Check sheet for the modelled part. Datum: model origin and axes. Units: mm. A direction names the side the tool comes from. Give positions to 0.01 mm unless a question says otherwise; leave off trailing zeros. Write each loop counter-clockwise with the first axis right and the second up, starting at its lowest first coordinate (ties: lowest second). Pieces come first, ordered by that corner, then holes. Notation, with made-up numbers: (75, 30) -> (115, 30) arc R18 ccw to (115, 52) -> close; hole circle Ø3 at (-15.75, -26). An arc over 180 degrees is marked (long way). Answer as a JSON object with one key per item and string values.
from build123d import *

# Parameters (mm, degrees)
SKETCH1_R           = 1.6
BOSS_EXTRUDE1_DEPTH = 7.5


with BuildPart() as part:
    # Sketch1 → Boss-Extrude1 (new body)
    with BuildSketch(Plane(origin=(0, 0, 0), x_dir=(1, 0, 0), z_dir=(0, 1, 0))):
        with BuildLine():
            Line((-5, 43.966606646), (-5, 44.520107817))
            ThreePointArc((-5, 44.520107817), (0, 44.8), (5, 44.520107817))
            Line((5, 44.520107817), (5, 43.966606646))
            ThreePointArc((5, 43.966606646), (31.289475068, 31.289475068), (43.966606646, 5))
            Line((43.966606646, 5), (44.520107817, 5))
            ThreePointArc((44.520107817, 5), (44.8, 0), (44.520107817, -5))
            Line((44.520107817, -5), (43.966606646, -5))
            ThreePointArc((43.966606646, -5), (31.289475068, -31.289475068), (5, -43.966606646))
            Line((5, -43.966606646), (5, -44.520107817))
            ThreePointArc((5, -44.520107817), (0, -44.8), (-5, -44.520107817))
            Line((-5, -44.520107817), (-5, -43.966606646))
            ThreePointArc((-5, -43.966606646), (-31.289475068, -31.289475068), (-43.966606646, -5))
            Line((-43.966606646, -5), (-44.520107817, -5))
            ThreePointArc((-44.520107817, -5), (-44.8, 0), (-44.520107817, 5))
            Line((-44.520107817, 5), (-43.966606646, 5))
            ThreePointArc((-43.966606646, 5), (-31.289475068, 31.289475068), (-5, 43.966606646))
        make_face()
        with Locations(Location((36.25, 0, 0), (0, 0, 270))):
            Circle(SKETCH1_R, mode=Mode.SUBTRACT)
        with Locations(Location((0, -36.25, 0), (0, 0, 270))):
            Circle(SKETCH1_R, mode=Mode.SUBTRACT)
        with Locations(Location((-36.25, 0, 0), (0, 0, 270))):
            Circle(SKETCH1_R, mode=Mode.SUBTRACT)
        with Locations(Location((0, 36.25, 0), (0, 0, 270))):
            Circle(SKETCH1_R, mode=Mode.SUBTRACT)
        with BuildLine():
            Line((33.430226046, 5), (36.586370413, 5))
            ThreePointArc((36.586370413, 5), (38.127746073, 5.725574218), (38.550739294, 7.375838926))
            ThreePointArc((38.550739294, 7.375838926), (36.262271651, 15.02032472), (32.474994896, 22.043983453))
            ThreePointArc((32.474994896, 22.043983453), (21.567115852, 32.79362764), (7.375838926, 38.550739294))
            ThreePointArc((7.375838926, 38.550739294), (5.725574218, 38.127746073), (5, 36.586370413))
            Line((5, 36.586370413), (5, 33.430226046))
            ThreePointArc((5, 33.430226046), (4.414213562, 32.016012484), (3, 31.430226046))
            Line((3, 31.430226046), (-3, 31.430226046))
            ThreePointArc((-3, 31.430226046), (-4.414213562, 32.016012484), (-5, 33.430226046))
            Line((-5, 33.430226046), (-5, 36.586370413))
            ThreePointArc((-5, 36.586370413), (-5.725574218, 38.127746073), (-7.375838926, 38.550739294))
            ThreePointArc((-7.375838926, 38.550739294), (-27.753941162, 27.753941162), (-38.550739294, 7.375838926))
            ThreePointArc((-38.550739294, 7.375838926), (-38.127746073, 5.725574218), (-36.586370413, 5))
            Line((-36.586370413, 5), (-33.430226046, 5))
            ThreePointArc((-33.430226046, 5), (-32.016012484, 4.414213562), (-31.430226046, 3))
            Line((-31.430226046, 3), (-31.430226046, -3))
            ThreePointArc((-31.430226046, -3), (-32.016012484, -4.414213562), (-33.430226046, -5))
            Line((-33.430226046, -5), (-36.586370413, -5))
            ThreePointArc((-36.586370413, -5), (-38.127746073, -5.725574218), (-38.550739294, -7.375838926))
            ThreePointArc((-38.550739294, -7.375838926), (-32.79362764, -21.567115852), (-22.043983453, -32.474994896))
            ThreePointArc((-22.043983453, -32.474994896), (-15.02032472, -36.262271651), (-7.375838926, -38.550739294))
            ThreePointArc((-7.375838926, -38.550739294), (-5.725574218, -38.127746073), (-5, -36.586370413))
            Line((-5, -36.586370413), (-5, -33.430226046))
            ThreePointArc((-5, -33.430226046), (-4.414213562, -32.016012484), (-3, -31.430226046))
            Line((-3, -31.430226046), (3, -31.430226046))
            ThreePointArc((3, -31.430226046), (4.414213562, -32.016012484), (5, -33.430226046))
            Line((5, -33.430226046), (5, -36.586370413))
            ThreePointArc((5, -36.586370413), (5.725574218, -38.127746073), (7.375838926, -38.550739294))
            ThreePointArc((7.375838926, -38.550739294), (27.753941162, -27.753941162), (38.550739294, -7.375838926))
            ThreePointArc((38.550739294, -7.375838926), (38.127746073, -5.725574218), (36.586370413, -5))
            Line((36.586370413, -5), (33.430226046, -5))
            ThreePointArc((33.430226046, -5), (32.016012484, -4.414213562), (31.430226046, -3))
            Line((31.430226046, -3), (31.430226046, 3))
            ThreePointArc((31.430226046, 3), (32.016012484, 4.414213562), (33.430226046, 5))
        make_face(mode=Mode.SUBTRACT)
    extrude(amount=BOSS_EXTRUDE1_DEPTH)


solid = part.part
1. Sectioned sample at C-C, the plane x = 18. Enter the section's corners in (y, z).
Determined:
{"outline": "(0, -40.42) -> (7.5, -40.42) -> (7.5, -34.88) -> (0, -34.88) -> close; (0, 34.88) -> (7.5, 34.88) -> (7.5, 40.42) -> (0, 40.42) -> close"}
2. Go/stop test with flat-tipped pins: P1, Ø3, axis at y = 1, z = -31, coming from the +X side; P2, Ø0.6, axis at x = -44.5, y = 2.5, coming from the -Z side; P3, Ø2.5, axis at x = 35.5, y = 4.5, coming from the +Z side; P4, Ø10, axis at x = 27, z = -13, coming from the -Y side. Record where each tip stops, or that it passes through.
Determined:
{"P1": "x = 32.98", "P2": "z = -5", "P3": "z = 28.02", "P4": "through"}
3. Sectioned sample at A-A, the plane x = 0. Enter the section's corners in (y, z), plus the area to 3 significant figures.
Determined:
{"outline": "(0, -44.8) -> (7.5, -44.8) -> (7.5, -37.85) -> (0, -37.85) -> close; (0, -34.65) -> (7.5, -34.65) -> (7.5, -31.43) -> (0, -31.43) -> close; (0, 31.43) -> (7.5, 31.43) -> (7.5, 34.65) -> (0, 34.65) -> close; (0, 37.85) -> (7.5, 37.85) -> (7.5, 44.8) -> (0, 44.8) -> close", "area": "153 mm^2"}
4. Sectioned sample at B-B, the plane z = 0. Enter the section's corners in (x, y).
Determined:
{"outline": "(-44.8, 0) -> (-37.85, 0) -> (-37.85, 7.5) -> (-44.8, 7.5) -> close; (-34.65, 0) -> (-31.43, 0) -> (-31.43, 7.5) -> (-34.65, 7.5) -> close; (31.43, 0) -> (34.65, 0) -> (34.65, 7.5) -> (31.43, 7.5) -> close; (37.85, 0) -> (44.8, 0) -> (44.8, 7.5) -> (37.85, 7.5) -> close"}
5. Mould release check, pull along X, two halves, no side actions. Record for faces 1 (the face through (31.583, 3.698, 30.994)), 2 (the face through (0, 4, 31.43)), 3 (the face through (1, 4, 35)), 4 (the face through (-31.583, 3.698, -30.994)): released by +X, released by -X, zero draft, split by the parting line, or undercut.
Determined:
{"face 1": "released by +X", "face 2": "undercut", "face 3": "undercut", "face 4": "released by -X"}
6. Access from +Z, -Z, +X, -X, +Y, -Y to the whole of each face (thin tool, end or side, straight path). Record for faces 5 (the face through (44.8, 3.7, -0.1)), 6 (the face through (-4.4, 3.7, -32)).
Determined:
{"face 5": "+X, +Y, -Y", "face 6": "+Y, -Y"}
7. Sectioned sample at D-D, the plane y = 6. State how many separate pieces and enclosed holes the cut face has, plus the area to 3 significant figures.
Determined:
{"separate pieces": "1", "enclosed holes": "5", "area": "1,610 mm^2"}
8. Scan lines: L1, parallel to X at y = 5.75, z = 0; L2, parallel to X at y = 6, z = 32.5; L3, parallel to Z at x = 35.5, y = 1. Record each from-to range of solid material in increasing order. Write a range as [from, to].
Determined:
{"L1": "[-44.8, -37.85], [-34.65, -31.43], [31.43, 34.65], [37.85, 44.8]", "L2": "[-30.03, -22.01], [-4.77, 4.77], [22.01, 30.03]", "L3": "[-26.42, -16.74], [-5, -1.41], [1.41, 5], [16.74, 26.42]"}
